Design review of the part built by this model. Coordinates are the model's own, in mm. Face numbers are marked on the shaded views. A direction names the side the tool comes from. Coordinates: 2 decimals unless noted, no trailing zeros. Loops run counter-clockwise (first coordinate to the right, second up) from the corner with the lowest first, then second, coordinate; pieces in that order, holes last. Notation, with made-up numbers: (-23, 68) - (33, 68) arc R26 ccw to (33, 94) - close; hole circle Ø5 at (88.25, 84.5). An arc over 180 degrees is marked (long way). Answer in a Markdown table with one row per item. Add a question column.
(1) We need section D-D, the plane x = 1. Write out the cut boundary in (y, z), plus the area to 3 significant figures.
(2) We need section C-C, the plane y = 4.25. Write out the cut boundary in (x, z), plus the area to 3 significant figures.
(3) To check wall thickness, follow L1, parallel to Y at x = -4, z = -14.5; L2, parallel to Z at x = -3, y = 0.5; L3, parallel to X at y = 6.75, z = -14. State the ranges of each line that lie inside material, in increasing order. Write a range as [from, to].
(4) We need section A-A, the plane y = 1. Write out the cut boundary in (x, z), plus the area to 3 significant figures.
(5) The part is to be moulded in two halves that separate along X. For the marked faces 1, 2, 3 and 4, say which applies: released by +X, released by -X, zero draft, split by the parting line, or undercut.
(6) For the marked faces 5, 6, 7, 8 and 9, list the 3-axis set-ups (+Z, -Z, +X, -X, +Y, -Y) from which the entire face can be reached by the end or side of a thin tool; tool diameter is ignored.
(7) Clearance check with flat-ended pins moving along their axes: pin 1 (4 mm diameter, centred on x = -5, z = -5, fed in from +Y); pin 2 (3 mm diameter, centred on y = 7, z = -11, fed in from -X); pin 3 (3 mm diameter, centred on y = 3.9, z = -3.9, fed in from +X). State where each tip first meets the part, or that it passes through.
(8) We need section B-B, the plane z = -1.25. Write out the cut boundary in (x, y), plus the area to 3 significant figures.
Autodesk Inventor part; units mm, degrees
ref_plane "YZ Plane" through (0, 0, 0) normal (1, 0, 0) x (0, 1, 0)
ref_plane "XZ Plane" through (0, 0, 0) normal (0, 1, 0) x (-1, 0, 0)
ref_plane "XY Plane" through (0, 0, 0) normal (0, 0, 1) x (1, 0, 0)
sketch "Sketch1" plane through (0, 0, 0) normal (0, 1, 0) x (-1, 0, 0)
  line L0 (0, 0) -> (7.7978, 0)
  line L1 (7.7978, 0) -> (7.7978, -15.5956)
  line L2 (7.7978, -15.5956) -> (0, -15.5956)
  line L3 (0, -15.5956) -> (0, 0)
  dimension "d0" = 7.7978
  dimension "d8" = 15.5956
extrude "Extrusion1" add sketch "Sketch1" along normal blind 3.236
sketch "Sketch2" plane through (0, 3.236, 0) normal (0, 1, 0) x (1, 0, 0)
  line L0 (0, 0) -> (0, 15.5956) construction
  line L1 (0, 0) -> (-3.8989, 0) construction
  line L2 (-3.8989, 0) -> (-3.8989, 3.8989) construction
  line L3 (-3.8989, 3.8989) -> (0, 3.8989) construction
  line L4 (0, 3.8989) -> (0, 0) construction
  circle A0 centre (-3.8989, 3.8989) radius 2.4498
  dimension "d11" = 3.8989
  dimension "d12" = 3.8989
  dimension "d13" = 4.8997
extrude "Extrusion2" add sketch "Sketch2" along normal blind 1.9837
pattern_linear "Rectangular Pattern1" count 2 spacing 7.7978 along (0, 0, -1) of "Extrusion2"
shell "Shell1" thickness 1.4732 removed faces 1 at (-2.5993, 0, -5.1985)
sketch "Sketch3" plane through (-6.3246, 1.7628, -1.4732) normal (0, -1, 0) x (1, 0, 0)
  circle A0 centre (2.4257, -2.4257) radius 2.4498 construction
  circle A1 centre (2.4257, -10.2235) radius 2.4498 construction
  circle A2 centre (2.4257, -2.4257) radius 0.9766 construction
  line L0 (2.4257, -2.4257) -> (2.4257, -10.2235) construction
  circle A3 centre (2.4257, -6.3246) radius 1.4491
  circle A4 centre (2.4257, -6.3246) radius 0.6198
  point P0 (6.3246, 1.4732)
  dimension "d20" = 1.2395
extrude "Extrusion3" add sketch "Sketch3" along normal up to surface (1.7628 mm away)
sketch "Sketch4" plane through (0, 0, 0) normal (1, 0, 0) x (0, 0, -1)
  line L0 (0, 0) -> (15.5956, 0)
  line L1 (15.5956, 0) -> (15.5956, 7.7978)
  line L2 (15.5956, 7.7978) -> (0, 7.7978)
  line L3 (0, 7.7978) -> (0, 0)
  dimension "d23" = 15.5956
  dimension "d24" = 7.7978
extrude "Extrusion4" add sketch "Sketch4" along normal blind 0.809
sketch "Sketch5" plane through (0.809, 0, 0) normal (1, 0, 0) x (0, 0, -1)
  line L0 (0, 0) -> (15.5956, 0) construction
  line L1 (0, 0) -> (3.8989, 0) construction
  line L2 (3.8989, 0) -> (3.8989, 3.8989) construction
  line L3 (3.8989, 3.8989) -> (0, 3.8989) construction
  line L4 (0, 3.8989) -> (0, 0) construction
  circle A0 centre (3.8989, 3.8989) radius 2.4498
  dimension "d27" = 3.8989
  dimension "d28" = 3.8989
  dimension "d29" = 4.8997
extrude "Extrusion5" add sketch "Sketch5" along normal blind 1.9837
sketch "Sketch6" plane through (2.7927, 3.8989, -3.8989) normal (1, 0, 0) x (0, 0, -1)
  circle A0 centre (0, 0) radius 2.4498 construction
  circle A1 centre (0, 0) radius 1.618
  point P0 (-3.8989, -3.8989)
  dimension "d32" = 3.236
extrude "Extrusion6" cut sketch "Sketch6" against normal blind 1.9837
pattern_linear "Rectangular Pattern2" count 2 spacing 7.7978 along (0, 0, -1) of "Extrusion6", "Extrusion5"
equation "\"d0\" = d1"
equation "\"d8\" = 2 * d1"
equation "\"d9\" = d2"
equation "\"d11\" = 0.5 * d1"
equation "\"d12\" = 0.5 * d1"
equation "\"d13\" = d4"
equation "\"d14\" = d5"
equation "\"d18\" = d1"
equation "\"d19\" = d6"
equation "\"d20\" = d7"
equation "\"d21\" = d5"
equation "\"d23\" = 2 * d1"
equation "\"d24\" = d1"
equation "\"d25\" = 0.25 * d2"
equation "\"d27\" = 0.5 * d1"
equation "\"d28\" = 0.5 * d1"
equation "\"d29\" = d4"
equation "\"d30\" = d5"
equation "\"d32\" = d2"
equation "\"d33\" = d5"
equation "\"d37\" = d1"
equation "\"d1\" = 7.7978"
equation "\"d2\" = 3.23596"
equation "\"d3\" = 9.60882"
equation "\"d4\" = 4.89966"
equation "\"d5\" = 1.98374"
equation "\"d6\" = 1.4732"
equation "\"d7\" = 1.23952"
properties part number "Two Sided Piece" material "ABS Plastic"
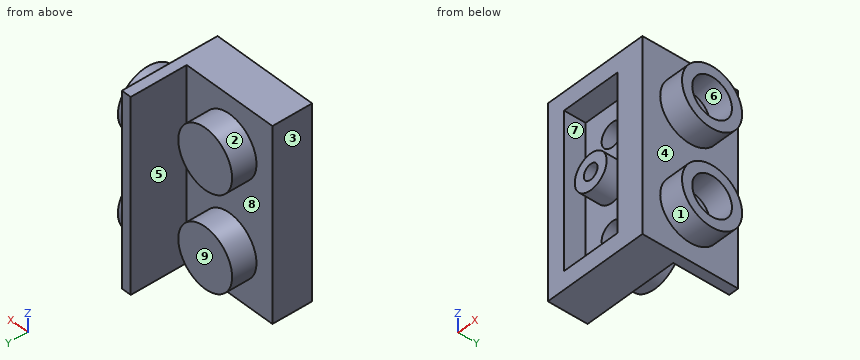
Responses:
| question | item | result |
|---|---|---|
| 1 | outline | circle Ø4.9 at (3.9, -11.7); circle Ø4.9 at (3.9, -3.9); hole circle Ø3.24 at (3.9, -11.7); hole circle Ø3.24 at (3.9, -3.9) |
| 1 | area | 21.3 mm2 |
| 2 | outline | circle Ø4.9 at (-3.9, -11.7); circle Ø4.9 at (-3.9, -3.9); (0, -15.6) - (0.81, -15.6) - (0.81, -14.12) - (2.79, -14.12) - (2.79, -13.28) - (0.81, -13.28) - (0.81, -10.12) - (2.79, -10.12) - (2.79, -9.27) - (0.81, -9.27) - (0.81, -6.32) - (2.79, -6.32) - (2.79, -5.48) - (0.81, -5.48) - (0.81, -2.32) - (2.79, -2.32) - (2.79, -1.47) - (0.81, -1.47) - (0.81, 0) - (0, 0) - close |
| 2 | area | 57.0 mm2 |
| 3 | L1 | y = [0, 3.24] |
| 3 | L2 | z = [-15.6, -14.12], [-8.93, -6.66], [-1.47, 0] |
| 3 | L3 | x = [0, 0.81] |
| 4 | outline | (-7.8, -15.6) - (0.81, -15.6) - (0.81, 0) - (-7.8, 0) - close; circle Ø2.9 at (-3.9, -7.8); hole (-6.32, -14.12) - (-1.47, -14.12) - (-1.47, -1.47) - (-6.32, -1.47) - close; hole circle Ø1.24 at (-3.9, -7.8) |
| 4 | area | 78.3 mm2 |
| 5 | face 1 | zero draft |
| 5 | face 2 | undercut |
| 5 | face 3 | released by -X |
| 5 | face 4 | released by +X |
| 6 | face 5 | +Z, -Z, +Y |
| 6 | face 6 | +X |
| 6 | face 7 | -Y |
| 6 | face 8 | +Y |
| 6 | face 9 | +Z, -Z, -X, +Y |
| 7 | pin 1 | stops at y = 5.22 |
| 7 | pin 2 | stops at x = 0 |
| 7 | pin 3 | stops at x = 0.81 |
| 8 | outline | (-7.8, 0) - (0.81, 0) - (0.81, 7.8) - (0, 7.8) - (0, 3.24) - (-7.8, 3.24) - close |
| 8 | area | 31.5 mm2 |
